Build history of the part. All positions in model axes, mm. A direction names the side the tool comes from. Round coordinates to 2 decimals unless told otherwise and drop trailing zeros. Write each loop counter-clockwise with the first axis right and the second up, starting at its lowest first coordinate (ties: lowest second). Pieces come first, ordered by that corner, then holes. Notation, with made-up numbers: (31, 22.25) -> (40, 22.25) arc R25 cw to (40, 59.25) -> close; hole circle Ø9 at (-8.5, 28). An arc over 180 degrees is marked (long way). Answer in a Markdown table with one row per item. Add a question column.
from build123d import *

# Parameters (mm, degrees)
PAD_DEPTH       = 29
POCKET_DEPTH    = 26
SKETCH004_R     = 4
PAD001_DEPTH    = 2
SKETCH005_R     = 1.25
POCKET001_DEPTH = 5
SKETCH006_R     = 1.25
POCKET002_DEPTH = 29
POCKET003_DEPTH = 1


with BuildPart() as part:
    # Sketch002 → Pad (new body)
    with BuildSketch(Plane.XY):
        with BuildLine():
            ThreePointArc((-41.415471, 40.271018), (-47.332493, 0), (-41.415471, -40.271018))
            ThreePointArc((-41.415471, -40.271018), (-40.693608, -41.300492), (-39.5, -41.695718))
            Line((-39.5, -41.695718), (39.5, -41.695718))
            ThreePointArc((39.5, -41.695718), (40.693608, -41.300492), (41.415471, -40.271018))
            ThreePointArc((41.415471, -40.271018), (47.332493, 0), (41.415471, 40.271018))
            ThreePointArc((41.415471, 40.271018), (40.693608, 41.300492), (39.5, 41.695718))
            Line((-39.5, 41.695718), (39.5, 41.695718))
            ThreePointArc((-39.5, 41.695718), (-40.693608, 41.300492), (-41.415471, 40.271018))
        make_face()
    extrude(amount=PAD_DEPTH)

    # Sketch003 → Pocket (cut)
    with BuildSketch(Plane.XY.offset(29)):
        with BuildLine():
            ThreePointArc((-39.924087, -38.205452), (-39.205905, -39.255214), (-38, -39.65966))
            Line((-38, -39.65966), (-33, -39.65966))
            Line((-33, -39.65966), (-33, -42.65966))
            Line((-33, -42.65966), (33, -42.65966))
            Line((33, -42.65966), (33, -39.65966))
            Line((33, -39.65966), (38, -39.65966))
            ThreePointArc((38, -39.65966), (39.205905, -39.255214), (39.924087, -38.205452))
            ThreePointArc((39.924087, -38.205452), (43.523931, -21.840329), (45.142785, -5.162336))
            ThreePointArc((45.142785, -5.162336), (44.579177, -3.987307), (43.291657, -3.785713))
            ThreePointArc((43.291657, 3.785713), (38, 0), (43.291657, -3.785713))
            ThreePointArc((43.291657, 3.785713), (44.579177, 3.987307), (45.142785, 5.162336))
            ThreePointArc((45.142785, 5.162336), (43.523931, 21.840329), (39.924087, 38.205452))
            ThreePointArc((39.924087, 38.205452), (39.205905, 39.255214), (38, 39.65966))
            Line((-38, 39.65966), (38, 39.65966))
            ThreePointArc((-38, 39.65966), (-39.205905, 39.255214), (-39.924087, 38.205452))
            ThreePointArc((-39.924087, 38.205452), (-43.523931, 21.840329), (-45.142785, 5.162336))
            ThreePointArc((-45.142785, 5.162336), (-44.579177, 3.987307), (-43.291657, 3.785713))
            ThreePointArc((-43.291657, -3.785713), (-38, 0), (-43.291657, 3.785713))
            ThreePointArc((-43.291657, -3.785713), (-44.579177, -3.987307), (-45.142785, -5.162336))
            ThreePointArc((-45.142785, -5.162336), (-43.523931, -21.840329), (-39.924087, -38.205452))
        make_face()
    extrude(amount=-POCKET_DEPTH, mode=Mode.SUBTRACT)

    # Sketch004 → Pad001 (new body)
    with BuildSketch(Plane.XY.offset(3)):
        with Locations((-32.55, 32.55)):
            Circle(SKETCH004_R)
        with Locations((32.55, 32.55)):
            Circle(SKETCH004_R)
        with Locations((32.55, -32.55)):
            Circle(SKETCH004_R)
        with Locations((-32.55, -32.55)):
            Circle(SKETCH004_R)
    extrude(amount=PAD001_DEPTH)

    # Sketch005 → Pocket001 (cut)
    with BuildSketch(Plane(origin=(0, 0, 0), x_dir=(1, 0, 0), z_dir=(0, 0, -1))):
        with Locations((-32.55, 32.55)):
            Circle(SKETCH005_R)
        with Locations((32.55, 32.55)):
            Circle(SKETCH005_R)
        with Locations((32.55, -32.55)):
            Circle(SKETCH005_R)
        with Locations((-32.55, -32.55)):
            Circle(SKETCH005_R)
    extrude(amount=-POCKET001_DEPTH, mode=Mode.SUBTRACT)

    # Sketch006 → Pocket002 (cut)
    with BuildSketch(Plane(origin=(0, 0, 0), x_dir=(1, 0, 0), z_dir=(0, 0, -1))):
        with Locations((-42, 0)):
            Circle(SKETCH006_R)
        with Locations((42, 0)):
            Circle(SKETCH006_R)
    extrude(amount=-POCKET002_DEPTH, mode=Mode.SUBTRACT)

    # Sketch008 → Pocket003 (cut)
    with BuildSketch(Plane.XY.offset(3)):
        with BuildLine():
            Line((-28.991378, 29.491378), (28.991378, 29.491378))
            ThreePointArc((29.491378, 28.991378), (29.344931, 29.344931), (28.991378, 29.491378))
            Line((29.491378, 28.991378), (29.491378, -28.991378))
            ThreePointArc((28.991378, -29.491378), (29.344931, -29.344931), (29.491378, -28.991378))
            Line((28.991378, -29.491378), (-28.991378, -29.491378))
            ThreePointArc((-29.491378, -28.991378), (-29.344931, -29.344931), (-28.991378, -29.491378))
            Line((-29.491378, -28.991378), (-29.491378, 28.991378))
            ThreePointArc((-28.991378, 29.491378), (-29.344931, 29.344931), (-29.491378, 28.991378))
        make_face()
    extrude(amount=-POCKET003_DEPTH, mode=Mode.SUBTRACT)


solid = part.part
(1) Saw through at B-B (x = -26). List the corners of the cut face in (y, z).
(2) Mould opens along X. For faces 1 (the face through (32, 31, 5)), 2 (the face through (-47.33, 0.57, 14.3)), 3 (the face through (3, 40, 29)) say: pulls with the +X half, pulls with the -X half, needs draft (parallel to the pull), parting line crosses it, or undercut.
(3) Drop flat-ended pins along their axis: P1, Ø2, axis at y = -8.5, z = 14.5, coming from the +X side; P2, Ø2, axis at x = 32.55, y = -32.55, coming from the +Z side; P3, Ø3, axis at x = -32.55, y = -32.55, coming from the +Z side; P4, Ø1, axis at y = -12.5, z = 17.5, coming from the -X side. Give the stop position or say it passes through.
(4) Which spindle directions (+Z, -Z, +X, -X, +Y, -Y) get a long thin tool onto all of the face, cutting with end or side? Do faces 4 (the face through (40.75, -0.05, 14.3)), 5 (the face through (-31, 0, 3)), 6 (the face through (33, -41, 16)). Say none if no direction does.
(5) Saw through at C-C (z = 27.25). Count the separate pieces of the cut face and the enclosed holes in it, plus the area to 4 significant figures.
(6) Probe line 1 along Y through (x, z) = (-32.55, 3.4); line 2 along Y through (x, z) = (32.55, 2.5); line 3 along Z through (x, y) = (-5, 15.5). List the from-to ranges inside material, lowest first.
(7) Saw through at A-A (y = 0). List the corners of the cut face in (x, z), plus the area to 3 significant figures.
(8) Saw through at D-D (y = 22.5). List the corners of the cut face in (x, z), plus the area to 3 significant figures.
Answer sheet:
| question | item | result |
|---|---|---|
| 1 | outline | (-41.7, 0) -> (41.7, 0) -> (41.7, 29) -> (39.66, 29) -> (39.66, 3) -> (29.49, 3) -> (29.49, 2) -> (-29.49, 2) -> (-29.49, 3) -> (-41.7, 3) -> close |
| 2 | face 1 | undercut |
| 2 | face 2 | pulls with the -X half |
| 2 | face 3 | needs draft |
| 3 | P1 | stops at x = 47.13 |
| 3 | P2 | passes through |
| 3 | P3 | stops at z = 5 |
| 3 | P4 | stops at x = -46.82 |
| 4 | face 4 | +Z, -Z |
| 4 | face 5 | +Z |
| 4 | face 6 | +Z, -Y |
| 5 | separate pieces | 1 |
| 5 | enclosed holes | 2 |
| 5 | area | 625.5 mm² |
| 6 | line 1 | y = -36.55 to -33.8, -31.3 to -28.55, 28.55 to 31.3, 33.8 to 36.55, 39.66 to 41.7 |
| 6 | line 2 | y = -41.7 to -33.8, -31.3 to 31.3, 33.8 to 41.7 |
| 6 | line 3 | z = 0 to 2 |
| 7 | outline | (-47.33, 0) -> (-43.25, 0) -> (-43.25, 29) -> (-47.33, 29) -> close; (-40.75, 0) -> (40.75, 0) -> (40.75, 29) -> (38, 29) -> (38, 3) -> (29.49, 3) -> (29.49, 2) -> (-29.49, 2) -> (-29.49, 3) -> (-38, 3) -> (-38, 29) -> (-40.75, 29) -> close; (43.25, 0) -> (47.33, 0) -> (47.33, 29) -> (43.25, 29) -> close |
| 7 | area | 565 mm² |
| 8 | outline | (-45.51, 0) -> (45.51, 0) -> (45.51, 29) -> (43.42, 29) -> (43.42, 3) -> (29.49, 3) -> (29.49, 2) -> (-29.49, 2) -> (-29.49, 3) -> (-43.42, 3) -> (-43.42, 29) -> (-45.51, 29) -> close |
| 8 | area | 323 mm² |
